Read the model definition and answer for the solid it produces. Units are mm, in the model's axes. A direction names the side the tool comes from. Give positions to 0.01 mm unless a question says otherwise; leave off trailing zeros. Order: outer loops, then holes, each group sorted by start corner. A loop starts at its lowest first (then second) coordinate and runs counter-clockwise, first axis right, second up. Notation, with made-up numbers: (-35, 22) - (3, 22) arc R37 ccw to (3, 59) - close; hole circle Ø10 at (-12, 89). An arc over 180 degrees is marked (long way). One line per item, written item: value. Start each with the question number.
```python
from build123d import *

# Parameters (mm, degrees)
SCHIZZO1_W                   = 60
SCHIZZO1_H                   = 7.2
SCHIZZO1_W_2                 = 19.125
SCHIZZO1_H_2                 = 5
ESTRUSIONE_ESTRUSIONE1_DEPTH = 40
SCHIZZO2_W                   = 11.375
SCHIZZO2_H                   = 5
SCHIZZO2_W_2                 = 2.075
SCHIZZO2_H_2                 = 1.1
SCHIZZO2_W_3                 = 2.05
TAGLIO_ESTRUSIONE1_DEPTH     = 61
SMUSSO1_SIZE                 = 0.75


with BuildPart() as part:
    # Schizzo1 → Estrusione-Estrusione1 (new body)
    with BuildSketch(Plane(origin=(0, 0, 0), x_dir=(0, 0, -1), z_dir=(1, 0, 0))):
        with Locations((30, 3.6)):
            Rectangle(SCHIZZO1_W, SCHIZZO1_H)
        with Locations((43.1875, 3.6)):
            Rectangle(SCHIZZO1_W_2, SCHIZZO1_H_2, mode=Mode.SUBTRACT)
        with Locations((16.8125, 3.6)):
            Rectangle(SCHIZZO1_W_2, SCHIZZO1_H_2, mode=Mode.SUBTRACT)
    extrude(amount=ESTRUSIONE_ESTRUSIONE1_DEPTH)

    # Schizzo2 → Taglio-Estrusione1 (cut, through all)
    with BuildSketch(Plane.XY):
        with Locations((10.6875, 2.5)):
            Rectangle(SCHIZZO2_W, SCHIZZO2_H)
        with Locations((29.3125, 2.5)):
            Rectangle(SCHIZZO2_W, SCHIZZO2_H)
        with Locations((15.3375, 6.65)):
            Rectangle(SCHIZZO2_W_2, SCHIZZO2_H_2)
        with Locations((8.275, 6.65)):
            Rectangle(SCHIZZO2_W_3, SCHIZZO2_H_2)
        with Locations((24.6625, 6.65)):
            Rectangle(SCHIZZO2_W_2, SCHIZZO2_H_2)
        with Locations((31.725, 6.65)):
            Rectangle(SCHIZZO2_W_3, SCHIZZO2_H_2)
    extrude(amount=-TAGLIO_ESTRUSIONE1_DEPTH, mode=Mode.SUBTRACT)

    # Smusso1
    smusso1_edges = [part.edges().sort_by_distance(p)[0] for p in [
        (40, 3.6, 0),
        (0, 3.6, 0),
        (0, 3.6, -60),
        (40, 3.6, -60),
    ]]
    chamfer(smusso1_edges, length=SMUSSO1_SIZE)


solid = part.part
```
1) The mould has two halves that part along Z. Classify faces 1 (the flat face through (12, 6.1, -17)), 2 (the flat face through (28, 6.1, -17)), 3 (the flat face through (20, 4, -60)), 4 (the flat face through (25, 6.1, -56)): +Z half, -Z half, draft (parallel to the pull), parting line (faces both ways), or undercut.
2) Section C-C on z = -40.5 is taken. Give the number of separate pieces and of enclosed holes in the cut face, plus the area to 3 significant figures.
3) Each of these flat-tipped pins is pushed along its axis until it touches: pin 1 (0.6 mm diameter, centred on x = 8, z = -29, fed in from +Y); pin 2 (3.5 mm diameter, centred on x = 29.5, z = -31, fed in from -Y). Where does it stop, or does it pass through?
4) For faces 5 (the flat face through (25, 6.1, -4)), 6 (the flat face through (16.375, 2, -30)), 7 (the flat face through (36, 7.2, -30)), 8 (the flat face through (36, 6.1, -43)), determine the directions among +Z, -Z, +X, -X, +Y, -Y from which every point of the face is accessible in a straight line to the end or side of a thin tool.
5) Section A-A on x = 20 is taken. Write down the section's boundary in (y, z) (3 decimals).
6) Find the intervals of material crossed by probe 1 along X at (y, z) = (1, -56) (3 decimals); probe 2 along Z at (x, y) = (3.5, 1.5) (3 decimals); probe 3 along Y at (x, z) = (30, -19.5), in increasing order. Write a range as from..to.
7) Section B-B on x = 24.5 is taken. Write down the section's boundary in (y, z) (3 decimals), plus the area to 3 significant figures.
Solved:
1. face 1: undercut
1. face 2: undercut
1. face 3: -Z half
1. face 4: draft
2. separate pieces: 8
2. enclosed holes: 0
2. area: 53.9 mm2
3. pin 1: stops at y = 6.1
3. pin 2: stops at y = 5
4. face 5: +Z, -Z, +Y
4. face 6: +Z, -Z, -Y
4. face 7: +Z, -Z, +X, -X, +Y
4. face 8: +X, -X
5. outline: (0, -60) - (7.2, -60) - (7.2, 0) - (0, 0) - close; hole (1.1, -52.75) - (6.1, -52.75) - (6.1, -33.625) - (1.1, -33.625) - close; hole (1.1, -26.375) - (6.1, -26.375) - (6.1, -7.25) - (1.1, -7.25) - close
6. probe 1: x = 0..5, 16.375..23.625, 35..40
6. probe 2: z = -60..-52.75, -33.625..-26.375, -7.25..0
6. probe 3: y = 6.1..7.2
7. outline: (5, -60) - (6.1, -60) - (6.1, -52.75) - (5, -52.75) - close; (5, -33.625) - (6.1, -33.625) - (6.1, -26.375) - (5, -26.375) - close; (5, -7.25) - (6.1, -7.25) - (6.1, 0) - (5, 0) - close
7. area: 23.9 mm2
